from build123d import *

# Parameters (mm, degrees)
SKETCH1_R           = 2.5
BOSS_EXTRUDE1_DEPTH = 70
SKETCH2_R           = 5
CUT_EXTRUDE1_DEPTH  = 60
SKETCH3_R           = 6
CUT_EXTRUDE2_DEPTH  = 65


with BuildPart() as part:
    # Sketch1 → Boss-Extrude1 (new body)
    with BuildSketch(Plane.XY):
        with BuildLine():
            Line((42.256479342, 32.363404542), (15.556670595, 0))
            Line((15.556670595, 0), (42.256479342, -32.363404542))
            ThreePointArc((42.256479342, -32.363404542), (40.636595458, -49.256479342), (23.743520658, -47.636595458))
            Line((23.743520658, -47.636595458), (0, -18.856570418))
            Line((0, -18.856570418), (-23.743520658, -47.636595458))
            ThreePointArc((-23.743520658, -47.636595458), (-40.636595458, -49.256479342), (-42.256479342, -32.363404542))
            Line((-42.256479342, -32.363404542), (-15.556670595, 0))
            Line((-15.556670595, 0), (-42.256479342, 32.363404542))
            ThreePointArc((-42.256479342, 32.363404542), (-40.636595458, 49.256479342), (-23.743520658, 47.636595458))
            Line((-23.743520658, 47.636595458), (0, 18.856570418))
            Line((0, 18.856570418), (23.743520658, 47.636595458))
            ThreePointArc((23.743520658, 47.636595458), (40.636595458, 49.256479342), (42.256479342, 32.363404542))
        make_face()
        with Locations((-33, 40)):
            Circle(SKETCH1_R, mode=Mode.SUBTRACT)
        with Locations((33, 40)):
            Circle(SKETCH1_R, mode=Mode.SUBTRACT)
        with Locations((-21, 21)):
            Circle(SKETCH1_R, mode=Mode.SUBTRACT)
        with Locations((21, 21)):
            Circle(SKETCH1_R, mode=Mode.SUBTRACT)
        with Locations((21, -21)):
            Circle(SKETCH1_R, mode=Mode.SUBTRACT)
        with Locations((-21, -21)):
            Circle(SKETCH1_R, mode=Mode.SUBTRACT)
        with Locations((-33, -40)):
            Circle(SKETCH1_R, mode=Mode.SUBTRACT)
        with Locations((33, -40)):
            Circle(SKETCH1_R, mode=Mode.SUBTRACT)
    extrude(amount=BOSS_EXTRUDE1_DEPTH)

    # Sketch2 → Cut-Extrude1 (cut)
    with BuildSketch(Plane.XY.offset(70)):
        with Locations((-21, -21)):
            Circle(SKETCH2_R)
        with Locations((-21, 21)):
            Circle(SKETCH2_R)
        with Locations((21, 21)):
            Circle(SKETCH2_R)
        with Locations((21, -21)):
            Circle(SKETCH2_R)
    extrude(amount=-CUT_EXTRUDE1_DEPTH, mode=Mode.SUBTRACT)

    # Sketch3 → Cut-Extrude2 (cut)
    with BuildSketch(Plane(origin=(0, 0, 0), x_dir=(-1, 0, 0), z_dir=(0, 0, -1))):
        with Locations((33, 40)):
            Circle(SKETCH3_R)
        with Locations((33, -40)):
            Circle(SKETCH3_R)
        with Locations((-33, 40)):
            Circle(SKETCH3_R)
        with Locations((-33, -40)):
            Circle(SKETCH3_R)
    extrude(amount=-CUT_EXTRUDE2_DEPTH, mode=Mode.SUBTRACT)


solid = part.part
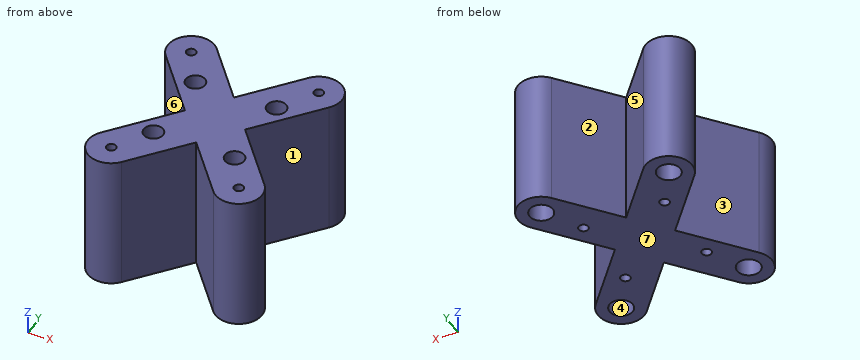
Geometry: final body of the model. Coordinates: model frame, mm. Face numbers are marked on the shaded views. A direction names the side the tool comes from. Give positions to 0.01 mm unless a question says otherwise; leave off trailing zeros. Write each loop counter-clockwise with the first axis right and the second up, starting at its lowest first coordinate (ties: lowest second). Pieces come first, ordered by that corner, then holes. Notation, with made-up numbers: M 0,-8 L 6,-8 A36 ccw 6,30 Z; hole C -2.75,-22.5 d11. An arc over 180 degrees is marked long. Answer in a Markdown table with one row per item. Add a question column.
(1) Mould query, pull axis X, two halves, no side actions, for the marked faces 5, 6 and 7. Classes: +X half, -X half, draft (parallel to the pull), parting line (faces both ways), or undercut.
(2) Section B-B on z = 7. State how many separate pieces and enclosed holes the cut face has, and give its area (3 significant figures).
(3) First-contact query: pin 1 (4 mm diameter, centred on y = -8, z = 8, fed in from -X); pin 2 (8 mm diameter, centred on y = 1.5, z = 30.5, fed in from +X); pin 3 (3.5 mm diameter, centred on x = -31, y = 37.5, fed in from -Z). Flat tips, straight axial feed; report the tip coordinate or a pass-through.
(4) Reachability of the marked faces 1, 2, 3 and 4 from +Z, -Z, +X, -X, +Y, -Y: full face, straight path, thin tool, end or side. Return the list, or none.
(5) Ray query, line 1 (X direction, y = 40, z = 67); line 2 (X direction, y = 18, z = 45); line 3 (Y direction, x = 20.5, z = 5). Return the intervals inside material, ascending.
(6) Section A-A on y = 40. Return loops of the section in (x, z), and give its area (3 significant figures).
(7) Section C-C on x = 21. Return loops of the section in (y, z), and give its area (3 significant figures).
Result set:
| question | item | result |
|---|---|---|
| 1 | face 5 | undercut |
| 1 | face 6 | -X half |
| 1 | face 7 | draft |
| 2 | separate pieces | 1 |
| 2 | enclosed holes | 8 |
| 2 | area | 4,770 mm^2 |
| 3 | pin 1 | stops at x = -23.81 |
| 3 | pin 2 | stops at x = 20.09 |
| 3 | pin 3 | stops at z = 65 |
| 4 | face 1 | +Z, -Z, +X |
| 4 | face 2 | +Z, -Z, +Y |
| 4 | face 3 | +Z, -Z, -X |
| 4 | face 4 | -Z |
| 5 | line 1 | x = -45 to -35.5, -30.5 to -17.44, 17.44 to 30.5, 35.5 to 45 |
| 5 | line 2 | x = -30.41 to -25, -17 to 17, 25 to 30.41 |
| 5 | line 3 | y = -43.71 to -23.45, -18.55 to -5.99, 5.99 to 18.55, 23.45 to 43.71 |
| 6 | outline | M -45,0 L -39,0 L -39,65 L -35.5,65 L -35.5,70 L -45,70 Z; M -30.5,65 L -27,65 L -27,0 L -17.44,0 L -17.44,70 L -30.5,70 Z; M 17.44,0 L 27,0 L 27,65 L 30.5,65 L 30.5,70 L 17.44,70 Z; M 35.5,65 L 39,65 L 39,0 L 45,0 L 45,70 L 35.5,70 Z |
| 6 | area | 2,250 mm^2 |
| 7 | outline | M -44.31,0 L -23.5,0 L -23.5,10 L -26,10 L -26,70 L -44.31,70 Z; M -18.5,0 L -6.6,0 L -6.6,70 L -16,70 L -16,10 L -18.5,10 Z; M 6.6,0 L 18.5,0 L 18.5,10 L 16,10 L 16,70 L 6.6,70 Z; M 23.5,0 L 44.31,0 L 44.31,70 L 26,70 L 26,10 L 23.5,10 Z |
| 7 | area | 3,980 mm^2 |
